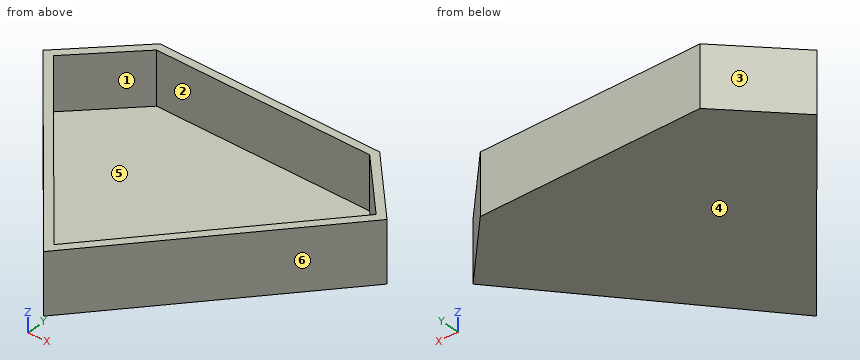
from build123d import *

# Parameters (mm, degrees)
F1_DEPTH = 10
F2_DEPTH = 10
F3_T     = 1.5
F4_R     = 5.8821297936
F5_DEPTH = 25.4


with BuildPart() as f1:
    # F0 (on Top) → F1 (new body)
    with BuildSketch(Plane.XY):
        Polygon((0, 16.2254609168), (-19.0141089261, 16.2254609168), (-26.4055486768, 8.4195453674), (0, -22.3205629736), (26.4055486768, 8.4195453674), (19.0141089261, 16.2254609168), align=None)
    extrude(amount=F1_DEPTH)

    # F0 (on Top) → F2 (join)
    with BuildSketch(Plane.XY):
        Polygon((-19.0141089261, 16.2254609168), (-20.2486366034, 19.1267747432), (-30.752800405, 8.3410236984), (-26.4055486768, 8.4195453674), align=None)
        Polygon((20.3608628362, 19.1267747432), (-20.2486366034, 19.1267747432), (-19.0141089261, 16.2254609168), (0, 16.2254609168), (19.0141089261, 16.2254609168), align=None)
        Polygon((30.752800405, 8.3410236984), (20.3608628362, 19.1267747432), (19.0141089261, 16.2254609168), (26.4055486768, 8.4195453674), align=None)
        Polygon((0, -27.7087166905), (30.752800405, 8.3410236984), (26.4055486768, 8.4195453674), (0, -22.3205629736), align=None)
        Polygon((-26.4055486768, 8.4195453674), (-30.752800405, 8.3410236984), (0, -27.7087166905), (0, -22.3205629736), align=None)
    extrude(amount=F2_DEPTH)

    # F3
    f3_openings = [f1.faces().sort_by_distance(p)[0] for p in [
        (0.008676, 1.980184, 10),
    ]]
    offset(amount=F3_T, openings=f3_openings, kind=Kind.INTERSECTION)

    # F4 (on face) → F5 (cut)
    with BuildSketch(Plane(origin=(0, 0, -1.5), x_dir=(1, 0, 0), z_dir=(0, 0, -1))):
        Circle(F4_R)
    extrude(amount=F5_DEPTH, mode=Mode.SUBTRACT)


solid = f1.part
For this review, take the finished solid that the model builds, in its own axes (mm). Face numbers are marked on the shaded views. A direction names the side the tool comes from. Round coordinates to 2 decimals unless told otherwise and drop trailing zeros. Loops run counter-clockwise (first coordinate to the right, second up) from the corner with the lowest first, then second, coordinate; pieces in that order, holes last. Notation, with made-up numbers: (72, 22) - (110, 22) arc R18 cw to (110, 28) - close; hole circle Ø5 at (14, 89). An arc over 180 degrees is marked (long way). One line per item, written item: value. Start each with the question number.
Item 1: Take a section at C-C (x = -3). Give the boundary of the cut face in (y, z).
Item 2: Take a section at A-A (z = 9). Give the boundary of the cut face in (x, y).
Item 3: The part is to be moulded in two halves that separate along Y. For the marked faces 1, 2, 3 and 4, say which applies: +Y half, -Y half, draft (parallel to the pull), parting line (faces both ways), or undercut.
Item 4: For L1, parallel to Z at x = -19, y = -4; L2, parallel to X at y = 1, z = 3; L3, parallel to Y at x = -7.5, z = 5, list the stretches that pass through material, from the lowest coordinate up.
Item 5: For the marked faces 5 and 6, list the 3-axis set-ups (+Z, -Z, +X, -X, +Y, -Y) from which the entire face can be reached by the end or side of a thin tool; tool diameter is ignored.
Item 6: Take a section at B-B (y = 7). Give the boundary of the cut face in (x, z).
Item 7: Clearance check with flat-ended pins moving along their axes: pin 1 Ø1.5 at (y, z) = (1, 6.5) entering from -X; pin 2 Ø3 at (x, z) = (0.5, 4) entering from -Y; pin 3 Ø6 at (y, z) = (-13, 7.5) entering from -X; pin 4 Ø8 at (x, y) = (19, -15) entering from +Z. State where each tip first meets the part, or that it passes through.
Answer below:
1. outline: (-26.5, -1.5) - (20.63, -1.5) - (20.63, 10) - (19.13, 10) - (19.13, 0) - (-24.19, 0) - (-24.19, 10) - (-26.5, 10) - close
2. outline: (-32.78, 8.41) - (0, -30.02) - (32.78, 8.4) - (21, 20.63) - (-20.88, 20.63) - close; hole (-30.75, 8.34) - (0, -27.71) - (30.75, 8.34) - (20.36, 19.13) - (-20.25, 19.13) - close
3. face 1: undercut
3. face 2: undercut
3. face 3: +Y half
3. face 4: draft
4. L1: z = -1.5 to 0
4. L2: x = -26.46 to -24.49, 24.49 to 26.46
4. L3: y = -21.23 to -18.92, 19.13 to 20.63
5. face 5: +Z
5. face 6: +Z, -Z, +X, -Y
6. outline: (-31.58, -1.5) - (31.58, -1.5) - (31.58, 10) - (29.61, 10) - (29.61, 0) - (-29.61, 0) - (-29.61, 10) - (-31.58, 10) - close
7. pin 1: stops at x = -27.1
7. pin 2: stops at y = -30.02
7. pin 3: stops at x = -17.08
7. pin 4: passes through
